Drawing for the job (mm, zero at the part's lowest x, y, z). A direction names the side the tool comes from. Coordinates: 2 decimals unless noted, no trailing zeros. Loops run counter-clockwise (first coordinate to the right, second up) from the corner with the lowest first, then second, coordinate; pieces in that order, holes last. Notation, with made-up numbers: (46, 76) - (62, 76) arc R28 cw to (62, 110) - close; hole circle Ø11 at (-15.75, -27.5). An arc over 180 degrees is marked (long way). Put each result on its own line as item: value.
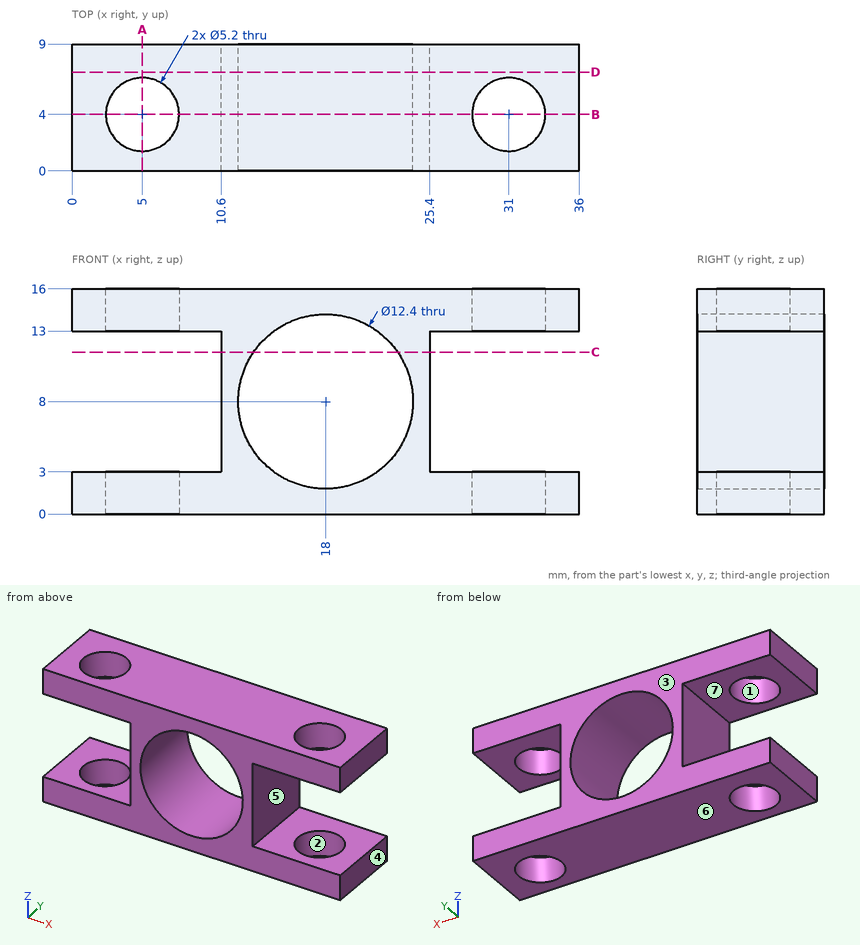
Q1. Slice it at C-C, the plane z = 11.5. Give the cut face in (x, y).
Determined:
outline: (10.6, 0) - (12.88, 0) - (12.88, 9) - (10.6, 9) - close; (23.12, 0) - (25.4, 0) - (25.4, 9) - (23.12, 9) - close
Q2. Slice it at D-D, the plane y = 7. Give the cut face in (x, z), then the cut area to 3 significant figures.
Determined:
outline: (0, 0) - (36, 0) - (36, 3) - (25.4, 3) - (25.4, 13) - (36, 13) - (36, 16) - (0, 16) - (0, 13) - (10.6, 13) - (10.6, 3) - (0, 3) - close; hole circle Ø12.4 at (18, 8)
area: 243 mm2
Q3. Tool access for the marked faces 5, 6 and 7: list every direction of +Z, -Z, +X, -X, +Y, -Y with a clear straight run to the whole face (end or side of a thin tool).
Determined:
face 5: +X, +Y, -Y
face 6: -Z, +X, -X, +Y, -Y
face 7: -X, +Y, -Y
Q4. Wall check: L1, parallel to Z at x = 8.5, y = 4.75; L2, parallel to Y at x = 5, z = 0.6; L3, parallel to X at y = 4.75, z = 12. Give the ranges that are in metal, low to high. Write a range as from..to.
Determined:
L1: 0..3, 13..16
L2: 0..1.4, 6.6..9
L3: 10.6..13.26, 22.74..25.4
Q5. Slice it at B-B, the plane y = 4. State how many separate pieces and enclosed holes the cut face has, then the cut area to 3 significant figures.
Determined:
separate pieces: 5
enclosed holes: 1
area: 181 mm2
Q6. Slice it at A-A, the plane x = 5. Give the cut face in (y, z), then the cut area to 3 significant figures.
Determined:
outline: (0, 0) - (1.4, 0) - (1.4, 3) - (0, 3) - close; (0, 13) - (1.4, 13) - (1.4, 16) - (0, 16) - close; (6.6, 0) - (9, 0) - (9, 3) - (6.6, 3) - close; (6.6, 13) - (9, 13) - (9, 16) - (6.6, 16) - close
area: 22.8 mm2
Q7. Pin check, flat tips, straight feed: pin 1 Ø4 at (x, z) = (27.5, 7) entering from -Y; pin 2 Ø4.5 at (y, z) = (6.5, 10) entering from -X; pin 3 Ø5 at (x, z) = (22, 9) entering from -Y; pin 4 Ø1.5 at (y, z) = (3, 9.5) entering from +X. Stop position of each tip, or through.
Determined:
pin 1: through
pin 2: x = 10.6
pin 3: y = 0
pin 4: x = 25.4
Q8. Mould opens along X. For the marked faces 1, 2, 3 and 4 say: +X half, -X half, draft (parallel to the pull), parting line (faces both ways), or undercut.
Determined:
face 1: undercut
face 2: undercut
face 3: draft
face 4: +X half
